```python
from build123d import *

# Parameters (mm, degrees)
F1_DEPTH = 914.4


with BuildPart() as f1:
    # F0 (on Front) → F1 (new body)
    with BuildSketch(Plane.XZ):
        Polygon((-13.0175, 20.6375), (-20.6375, 20.6375), (-20.6375, -20.6375), (20.6375, -20.6375), (20.6375, 20.6375), (13.0175, 20.6375), (13.0175, 10.4775), (14.2875, 10.4775), (14.2875, 19.3675), (19.3675, 19.3675), (19.3675, -19.3675), (-19.3675, -19.3675), (-19.3675, 19.3675), (-14.2875, 19.3675), (-14.2875, 10.4775), (-13.0175, 10.4775), align=None)
    extrude(amount=-F1_DEPTH)


solid = f1.part
```
Here's how the part is built. I have some questions about the finished solid (model axes, mm). A direction names the side the tool comes from. Coordinates: 2 decimals unless noted, no trailing zeros. Loops run counter-clockwise (first coordinate to the right, second up) from the corner with the lowest first, then second, coordinate; pieces in that order, holes last. Notation, with made-up numbers: (73.5, 0.25) -> (78.5, 0.25) arc R16 ccw to (78.5, 24.25) -> close; hole circle Ø10 at (13, 42). An arc over 180 degrees is marked (long way). Return JSON: item names as keys, results as strings.
1) Thinking about a two-plate mould opening in Z: for faces 1 (the face through (-19.368, 451, 0)), 2 (the face through (0, 451, -20.638)), 3 (the face through (-20.638, 451, 0)), which applies, +Z half, -Z half, draft (parallel to the pull), parting line (faces both ways), or undercut?
Results below:
{"face 1": "undercut", "face 2": "-Z half", "face 3": "draft"}
2) For faces 4 (the face through (19.368, 451, 0)), 5 (the face through (20.638, 451, 0)), which set-ups out of +Z, -Z, +X, -X, +Y, -Y let a thin tool reach every point of the face, with its end or its side?
Results below:
{"face 4": "+Y, -Y", "face 5": "+Z, -Z, +X, +Y, -Y"}
3) I need wall thicknesses on line 1 (X direction, y = 468, z = 18); line 2 (X direction, y = 213, z = -2). Which ranges of each line are inside material? Lowest first, please. Write a range as from..to.
Results below:
{"line 1": "-20.64..-19.37, -14.29..-13.02, 13.02..14.29, 19.37..20.64", "line 2": "-20.64..-19.37, 19.37..20.64"}
4) If we section it at A-A, the plane z = -3: Write out the boundary of the cut face in (x, y).
Results below:
{"outline": "(-20.64, 0) -> (-19.37, 0) -> (-19.37, 914.4) -> (-20.64, 914.4) -> close; (19.37, 0) -> (20.64, 0) -> (20.64, 914.4) -> (19.37, 914.4) -> close"}
5) If we section it at B-B, the plane y = 128.5: Write out the boundary of the cut face in (x, z), then the cut area to 3 significant figures.
Results below:
{"outline": "(-20.64, -20.64) -> (20.64, -20.64) -> (20.64, 20.64) -> (13.02, 20.64) -> (13.02, 10.48) -> (14.29, 10.48) -> (14.29, 19.37) -> (19.37, 19.37) -> (19.37, -19.37) -> (-19.37, -19.37) -> (-19.37, 19.37) -> (-14.29, 19.37) -> (-14.29, 10.48) -> (-13.02, 10.48) -> (-13.02, 20.64) -> (-20.64, 20.64) -> close", "area": "193 mm²"}
6) If we section it at C-C, the plane x = -1: Write out the boundary of the cut face in (y, z), then the cut area to 3 significant figures.
Results below:
{"outline": "(0, -20.64) -> (914.4, -20.64) -> (914.4, -19.37) -> (0, -19.37) -> close", "area": "1,160 mm²"}
7) Will these pins go through, and if not, where does the flat tip stop? pin 1 (6 mm diameter, centred on x = -14.5, z = -15, fed in from -Y); pin 2 (8 mm diameter, centred on x = 5.5, y = 301.5, fed in from +Z).
Results below:
{"pin 1": "through", "pin 2": "z = -19.37"}
